Source: CAD feature listing. Evaluate the final solid. Frame: model axes, mm. Round coordinates to 2 decimals unless told otherwise and drop trailing zeros. Loops run counter-clockwise (first coordinate to the right, second up) from the corner with the lowest first, then second, coordinate; pieces in that order, holes last. Notation, with made-up numbers: M 64,20 L 119,20 A13 ccw 119,27 Z; hole C -1,87 d11. An arc over 180 degrees is marked long. Answer as a JSON object with one key per item and string values.
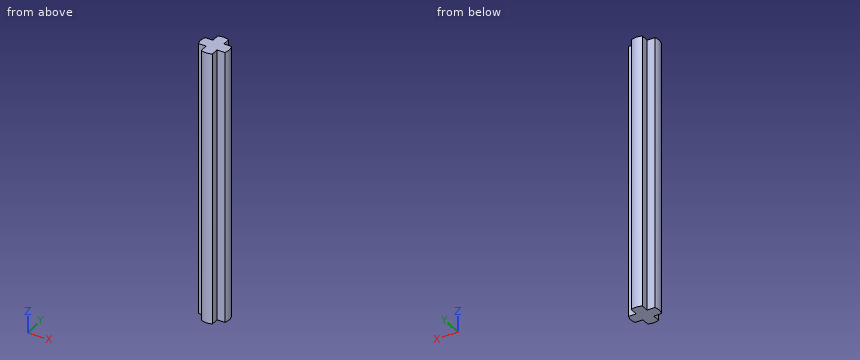
from build123d import *

# Parameters (mm, degrees)
BOSS_EXTRUDE1_DEPTH = 45


with BuildPart() as part:
    # Sketch1 → Boss-Extrude1 (new body)
    with BuildSketch(Plane.XY):
        with BuildLine():
            Line((-0.9, 2.170829335), (-0.9, 0.9))
            Line((-0.9, 0.9), (-2.170829335, 0.9))
            ThreePointArc((-2.170829335, 0.9), (-2.35, 0), (-2.170829335, -0.9))
            Line((-2.170829335, -0.9), (-0.9, -0.9))
            Line((-0.9, -0.9), (-0.9, -2.170829335))
            ThreePointArc((-0.9, -2.170829335), (0, -2.35), (0.9, -2.170829335))
            Line((0.9, -2.170829335), (0.9, -0.9))
            Line((0.9, -0.9), (2.170829335, -0.9))
            ThreePointArc((2.170829335, -0.9), (2.35, 0), (2.170829335, 0.9))
            Line((2.170829335, 0.9), (0.9, 0.9))
            Line((0.9, 0.9), (0.9, 2.170829335))
            ThreePointArc((0.9, 2.170829335), (0, 2.35), (-0.9, 2.170829335))
        make_face()
    extrude(amount=BOSS_EXTRUDE1_DEPTH)


solid = part.part
Item 1: Contact query for flat-ended pins moving along their axis: pin 1 Ø1 at (y, z) = (-1.5, 33) entering from -X; pin 2 Ø0.6 at (y, z) = (1.5, 14.5) entering from +X; pin 3 Ø1.4 at (x, z) = (1.5, 16.5) entering from +Y. Output: stop coordinate, or through.
Answer sheet:
{"pin 1": "stops at x = -0.9", "pin 2": "stops at x = 0.9", "pin 3": "stops at y = 2.21"}
Item 2: Section A-A on z = 4.5. Return the cut outline in (x, y), then the cut area to 3 significant figures.
Answer sheet:
{"outline": "M -2.17,-0.9 L -0.9,-0.9 L -0.9,-2.17 A2.35 ccw 0.9,-2.17 L 0.9,-0.9 L 2.17,-0.9 A2.35 ccw 2.17,0.9 L 0.9,0.9 L 0.9,2.17 A2.35 ccw -0.9,2.17 L -0.9,0.9 L -2.17,0.9 A2.35 ccw Z", "area": "13.3 mm²"}
Item 3: Line query: probe 1 along Y at (x, z) = (-1.25, 3.5); probe 2 along X at (y, z) = (0.15, 30). Output: solid intervals per line, ascending. Write a range as from..to.
Answer sheet:
{"probe 1": "y = -0.9..0.9", "probe 2": "x = -2.35..2.35"}
Item 4: Section B-B on y = -1.55. Return the cut outline in (x, z).
Answer sheet:
{"outline": "M -0.9,0 L 0.9,0 L 0.9,45 L -0.9,45 Z"}
